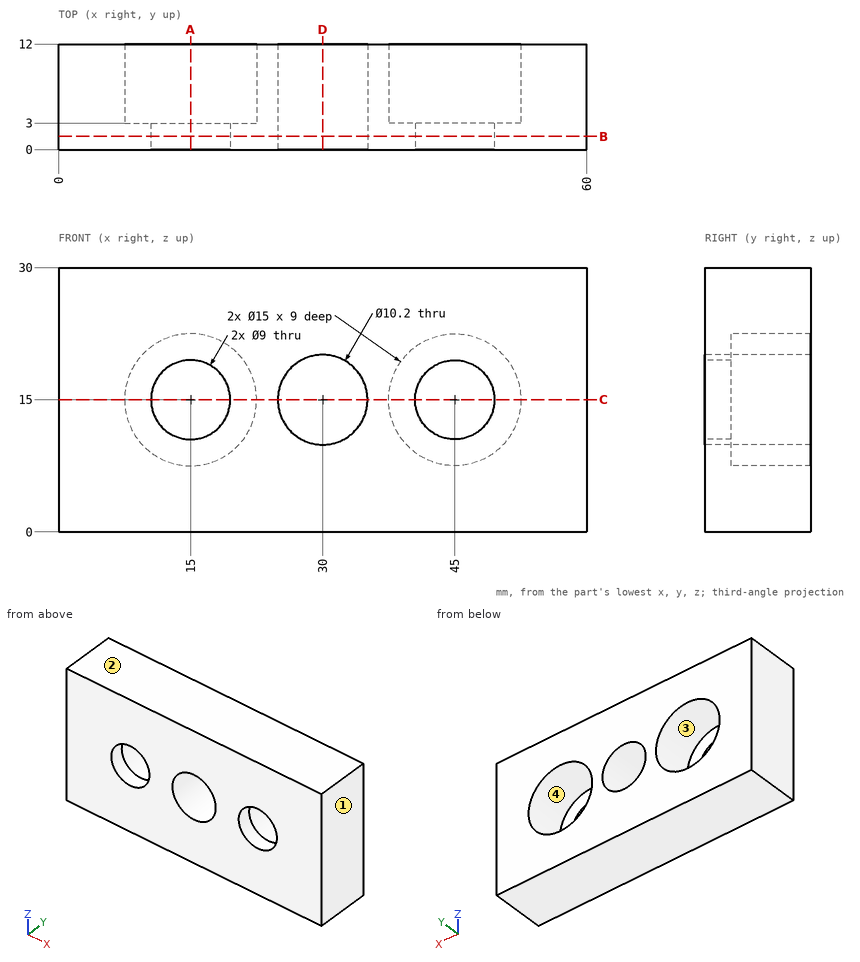
For this review, use the dimensioned drawing (mm, ordinates from the lowest corner) and the shaded views. Give positions to 0.01 mm unless a question says otherwise; leave off trailing zeros. Loops run counter-clockwise (first coordinate to the right, second up) from the corner with the lowest first, then second, coordinate; pieces in that order, holes last. Notation, with made-up numbers: (19.5, 62) -> (45.5, 62) arc R7 cw to (45.5, 74) -> close; hole circle Ø1 at (-6, -29). An arc over 180 degrees is marked (long way). One line per question, with ' | ' between items. Start each with the question number.
(1) We need section D-D (x = 30). State the section outline as (y, z) points, and give its area (3 significant figures).
(2) We need section A-A (x = 15). State the section outline as (y, z) points.
(3) For line 1 (X direction, y = 6, z = 12.5); line 2 (Z direction, x = 45, y = 2.25); line 3 (Z direction, x = 45, y = 7.75), list the stretches that pass through material, from the lowest coordinate up.
(4) Draft analysis for pull direction Z (two halves, no side actions). For the marked faces 1, 2, 3 and 4, state which applies: +Z half, -Z half, draft (parallel to the pull), parting line (faces both ways), or undercut.
(5) Insertion check: P1, Ø8, axis at x = 15, z = 15, coming from the +Y side; P2, Ø10, axis at x = 47.5, z = 10.5, coming from the -Y side; P3, Ø10.5, axis at x = 45, z = 15, coming from the +Y side. Each pin has a flat end and moves straight along its axis. Give the tip position at first contact, or say it passes through.
(6) We need section C-C (z = 15). State the section outline as (x, y) points, and give its area (3 significant figures).
(7) We need section B-B (y = 1.5). State the section outline as (x, z) points.
The answers:
1) outline: (0, 0) -> (12, 0) -> (12, 9.9) -> (0, 9.9) -> close; (0, 20.1) -> (12, 20.1) -> (12, 30) -> (0, 30) -> close | area: 238 mm^2
2) outline: (0, 0) -> (12, 0) -> (12, 7.5) -> (3, 7.5) -> (3, 10.5) -> (0, 10.5) -> close; (0, 19.5) -> (3, 19.5) -> (3, 22.5) -> (12, 22.5) -> (12, 30) -> (0, 30) -> close
3) line 1: x = 0 to 7.93, 22.07 to 25.55, 34.45 to 37.93, 52.07 to 60 | line 2: z = 0 to 10.5, 19.5 to 30 | line 3: z = 0 to 7.5, 22.5 to 30
4) face 1: draft | face 2: +Z half | face 3: undercut | face 4: undercut
5) P1: passes through | P2: stops at y = 0 | P3: stops at y = 3
6) outline: (0, 0) -> (10.5, 0) -> (10.5, 3) -> (7.5, 3) -> (7.5, 12) -> (0, 12) -> close; (19.5, 0) -> (24.9, 0) -> (24.9, 12) -> (22.5, 12) -> (22.5, 3) -> (19.5, 3) -> close; (35.1, 0) -> (40.5, 0) -> (40.5, 3) -> (37.5, 3) -> (37.5, 12) -> (35.1, 12) -> close; (49.5, 0) -> (60, 0) -> (60, 12) -> (52.5, 12) -> (52.5, 3) -> (49.5, 3) -> close | area: 274 mm^2
7) outline: (0, 0) -> (60, 0) -> (60, 30) -> (0, 30) -> close; hole circle Ø9 at (15, 15); hole circle Ø10.2 at (30, 15); hole circle Ø9 at (45, 15)
